Design review of the part built by this model. Coordinates are the model's own, in mm. A direction names the side the tool comes from. Round coordinates to 2 decimals unless told otherwise and drop trailing zeros. Loops run counter-clockwise (first coordinate to the right, second up) from the corner with the lowest first, then second, coordinate; pieces in that order, holes last. Notation, with made-up numbers: (-19.5, -21) -> (10.5, -21) arc R25 cw to (10.5, 15) -> close; hole circle Ø1 at (-7, 18.5). An arc over 180 degrees is marked (long way). Answer as CSV lines item,"result". Start each with the question number.
(1) For P1, Ø2, axis at x = -22, y = 11.5, coming from the -Z side, flat-tipped, find the tip position at first contact; note if it passes through.
(2) Machinability: for faces 1 (the face through (38.768, 2, -2)), 2 (the face through (40, 6.541, -2)), 3 (the face through (40.768, 3, -2)), which of the approach directions +Z, -Z, +X, -X, +Y, -Y give a long, thin tool a straight path to every point of the face, cutting with its end or side? Answer none if there is none.
(3) Draft analysis for pull direction Y (two halves, no side actions). For faces 4 (the face through (-1, 4.541, -2)), 5 (the face through (80, 3, 0)), 6 (the face through (57, 5, -5)), state which applies: +Y half, -Y half, draft (parallel to the pull), parting line (faces both ways), or undercut.
(4) To check wall thickness, follow line 1 (Y direction, x = 48.5, z = -1); line 2 (Y direction, x = -17, z = -0.5); line 3 (Z direction, x = 26, y = 12.5). State the ranges of each line that lie inside material, in increasing order. Write a range as from..to.
(5) Take a section at A-A, the plane z = -2.5. Write out the cut boundary in (x, y).
(6) Take a section at C-C, the plane x = 96.5. Write out the cut boundary in (y, z).
(7) Take a section at B-B, the plane x = 5. Write out the cut boundary in (y, z), and give its area (3 significant figures).
from build123d import *

# Parameters (mm, degrees)
ESBO_O1_W                = 160
ESBO_O1_H                = 2
ESBO_O1_W_2              = 80
RESSALTO_EXTRUS_O1_DEPTH = 5
ESBO_O1_3_W              = 160
ESBO_O1_3_H              = 7.85
ESBO_O1_3_W_2            = 80
ESBO_O1_3_H_2            = 3.5
ESBO_O1_3_H_3            = 2
RESSALTO_EXTRUS_O2_DEPTH = 2


with BuildPart() as part:
    # Esbo_o1 → Ressalto-extrus_o1 (new body)
    with BuildSketch(Plane.XY):
        with Locations((40.767792431, 15.391143911)):
            Rectangle(ESBO_O1_W, ESBO_O1_H)
        with Locations((40.767792431, 5.541143911)):
            Rectangle(ESBO_O1_W, ESBO_O1_H)
        with Locations((80.767792431, 0.041143911)):
            Rectangle(ESBO_O1_W_2, ESBO_O1_H)
        Polygon((40.767792431, 4.541143911), (38.767792431, 4.541143911), (38.767792431, -0.958856089), (40.767792431, -0.958856089), (40.767792431, 1.041143911), align=None)
    extrude(amount=-RESSALTO_EXTRUS_O1_DEPTH)

    # Esbo_o1_3 → Ressalto-extrus_o2 (add)
    with BuildSketch(Plane.XY):
        with Locations((40.767792431, 10.466143911)):
            Rectangle(ESBO_O1_3_W, ESBO_O1_3_H)
        with Locations((80.767792431, 2.791143911)):
            Rectangle(ESBO_O1_3_W_2, ESBO_O1_3_H_2)
        with Locations((40.767792431, 15.391143911)):
            Rectangle(ESBO_O1_3_W, ESBO_O1_3_H_3)
        with Locations((40.767792431, 5.541143911)):
            Rectangle(ESBO_O1_3_W, ESBO_O1_3_H_3)
        with Locations((80.767792431, 0.041143911)):
            Rectangle(ESBO_O1_3_W_2, ESBO_O1_3_H_3)
        Polygon((40.767792431, 4.541143911), (38.767792431, 4.541143911), (38.767792431, -0.958856089), (40.767792431, -0.958856089), (40.767792431, 1.041143911), align=None)
    extrude(amount=RESSALTO_EXTRUS_O2_DEPTH)


solid = part.part
The answers:
1,P1,"z = 0"
2,face 1,"+Z, -Z, -X, -Y"
2,face 2,"-Z, +X, -X"
2,face 3,"-Z, +X"
3,face 4,"-Y half"
3,face 5,"undercut"
3,face 6,"draft"
4,line 1,"-0.96..1.04, 4.54..6.54, 14.39..16.39"
4,line 2,"4.54..6.54, 14.39..16.39"
4,line 3,"0..2"
5,outline,"(-39.23, 4.54) -> (38.77, 4.54) -> (38.77, -0.96) -> (120.77, -0.96) -> (120.77, 1.04) -> (40.77, 1.04) -> (40.77, 4.54) -> (120.77, 4.54) -> (120.77, 6.54) -> (-39.23, 6.54) -> close; (-39.23, 14.39) -> (120.77, 14.39) -> (120.77, 16.39) -> (-39.23, 16.39) -> close"
6,outline,"(-0.96, -5) -> (1.04, -5) -> (1.04, 0) -> (4.54, 0) -> (4.54, -5) -> (6.54, -5) -> (6.54, 0) -> (14.39, 0) -> (14.39, -5) -> (16.39, -5) -> (16.39, 2) -> (-0.96, 2) -> close"
7,outline,"(4.54, -5) -> (6.54, -5) -> (6.54, 0) -> (14.39, 0) -> (14.39, -5) -> (16.39, -5) -> (16.39, 2) -> (4.54, 2) -> close"
7,area,"43.7 mm²"
